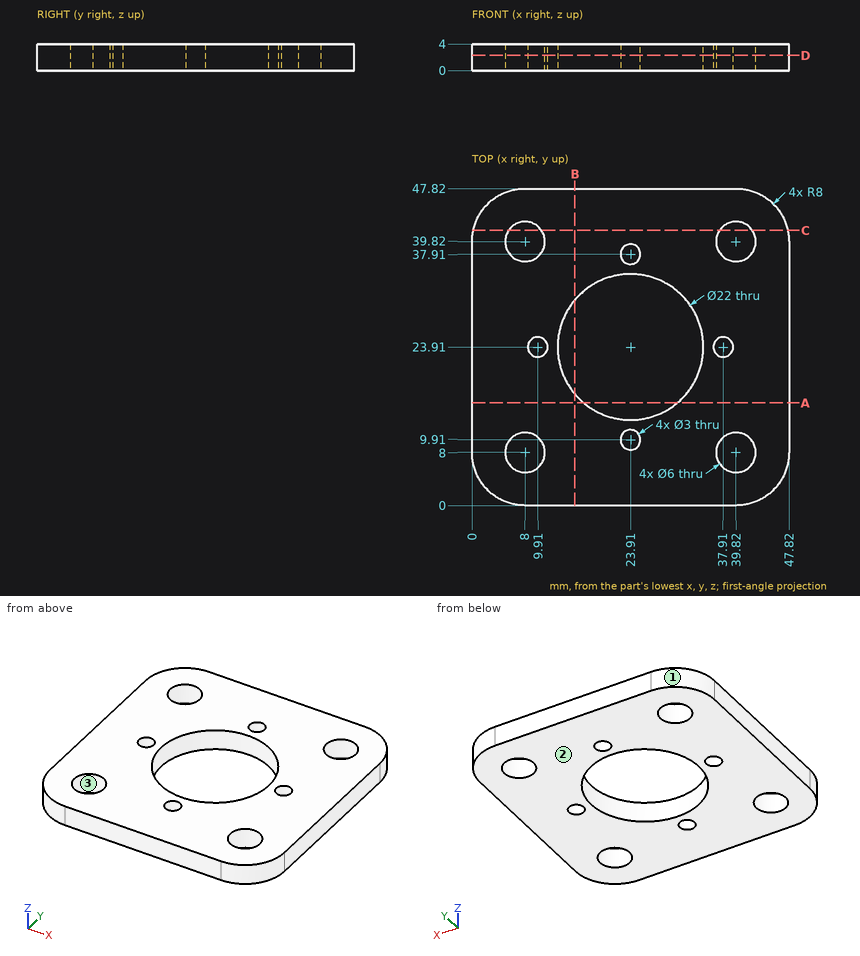
Part print with two shaded views. Sizes in mm from the minimum x, y, z corner. Coordinates: 2 decimals unless noted, no trailing zeros. Order: outer loops, then holes, each group sorted by start corner. A loop starts at its lowest first (then second) coordinate and runs counter-clockwise, first axis right, second up. Notation, with made-up numbers: M 55,79 L 103,79 A8 cw 103,89 Z; hole C 42.25,-19.75 d1. An arc over 180 degrees is marked long. Use a Markdown table: item, result.
(1) Probe L1, parallel to Y at x = 8, z = 3; L2, parallel to X at y = 23, z = 0.65; L3, parallel to X at y = 5.5, z = 2. List the from-to ranges inside material, lowest first.
A:
| item | result |
|---|---|
| L1 | y = 0 to 5, 11 to 36.82, 42.82 to 47.82 |
| L2 | x = 0 to 8.72, 11.1 to 12.95, 34.87 to 36.72, 39.1 to 47.82 |
| L3 | x = 0.4 to 6.34, 9.66 to 38.16, 41.48 to 47.42 |
(2) Pull direction X, two halves, no side cores. Call the marked faces 1, 2 and 3: released by +X, released by -X, zero draft, split by the parting line, or undercut.
A:
| item | result |
|---|---|
| face 1 | released by -X |
| face 2 | zero draft |
| face 3 | undercut |
(3) Cut at D-D on z = 2.3. State how many separate pieces and enclosed holes the cut face has, then the cut area to 3 significant figures.
A:
| item | result |
|---|---|
| separate pieces | 1 |
| enclosed holes | 9 |
| area | 1,710 mm^2 |
(4) Flat gauge pins, fed straight in: pin 1 (2 mm diameter, centred on y = 43, z = 3, fed in from +X); pin 2 (3.5 mm diameter, centred on x = 23.91, y = 9.91, fed in from -Z). Where does each tip first touch, or does it go through?
A:
| item | result |
|---|---|
| pin 1 | stops at x = 47.52 |
| pin 2 | stops at z = 0 |
(5) Cut at C-C on y = 41.5. Write the cut outline in (x, z) (1 decimal), then the cut area to 3 significant figures.
A:
| item | result |
|---|---|
| outline | M 0.2,0 L 5.5,0 L 5.5,4 L 0.2,4 Z; M 10.5,0 L 37.3,0 L 37.3,4 L 10.5,4 Z; M 42.3,0 L 47.6,0 L 47.6,4 L 42.3,4 Z |
| area | 150 mm^2 |
(6) Cut at A-A on y = 15.5. Write the cut outline in (x, z), then the cut area to 3 significant figures.
A:
| item | result |
|---|---|
| outline | M 0,0 L 16.82,0 L 16.82,4 L 0,4 Z; M 31,0 L 47.82,0 L 47.82,4 L 31,4 Z |
| area | 135 mm^2 |
